Autodesk Inventor part; units mm, degrees
ref_plane "YZ Plane" through (0, 0, 0) normal (1, 0, 0) x (0, 1, 0)
ref_plane "XZ Plane" through (0, 0, 0) normal (0, 1, 0) x (-1, 0, 0)
ref_plane "XY Plane" through (0, 0, 0) normal (0, 0, 1) x (1, 0, 0)
sketch "Sketch1" plane through (0, 0, 0) normal (0, 0, 1) x (1, 0, 0)
  line L0 (-17.23, 12.6) -> (17.23, 12.6)
  line L1 (17.23, 12.6) -> (17.23, -12.6)
  line L2 (17.23, -12.6) -> (-17.23, -12.6)
  line L3 (-17.23, -12.6) -> (-17.23, 12.6)
  point P0 (0, 0)
  dimension "d0" = 17.23
  dimension "d1" = 34.46
  dimension "d2" = 12.6
  dimension "d3" = 25.2
extrude "Plate1" add sketch "Sketch1" along normal blind 0.5
sketch "Sketch4" plane through (-16.73, -12.6, 0) normal (-1, 0, 0) x (0, -1, 0)
  line L0 (-25.2, 0) -> (0, 0)
  line L1 (0, 0) -> (0, 8.75)
  line L2 (0, 8.75) -> (-25.2, 8.75)
  line L3 (-25.2, 8.75) -> (-25.2, 0)
edge flange "Flange1" height 8.75 angle 90 thickness 0.5 bend radius 0.5 thickness toward (-1, 0, 0) relief straight relief width 0.5 relief depth 0.25 edges at (-17.23, 0, 0.5) wall of the first edge with corners at (-16.73, 12.6, 0) (-16.73, -12.6, 0) (-16.73, -12.6, 8.75) (-16.73, 12.6, 8.75)
bend "Bend1"
corner "Corner1"
sketch "Sketch5" plane through (16.73, 12.6, 0) normal (1, 0, 0) x (0, 1, 0)
  line L0 (-25.2, 0) -> (0, 0)
  line L1 (0, 0) -> (0, 8.75)
  line L2 (0, 8.75) -> (-25.2, 8.75)
  line L3 (-25.2, 8.75) -> (-25.2, 0)
edge flange "Flange2" height 8.75 angle 90 thickness 0.5 bend radius 0.5 thickness toward (1, 0, 0) relief straight relief width 0.5 relief depth 0.25 edges at (17.23, 0, 0.5) wall of the first edge with corners at (16.73, -12.6, 0) (16.73, 12.6, 0) (16.73, 12.6, 8.75) (16.73, -12.6, 8.75)
bend "Bend2"
corner "Corner2"
sketch "Sketch6" plane through (0, 0, 0.5) normal (0, 0, 1) x (1, 0, 0)
  circle A0 centre (0, 0) radius 4
  circle A1 centre (0, 8.04) radius 1.65
  circle A2 centre (0, -8.04) radius 1.65
  circle A3 centre (8.04, 0) radius 1.65
  circle A4 centre (-8.04, 0) radius 1.65
  line L0 (16.23, -12.6) -> (-16.23, -12.6)
  line L1 (-16.23, 12.6) -> (16.23, 12.6)
  dimension "d26" = 3.3
  dimension "d27" = 8
  dimension "d29" = 4.56
  dimension "d30" = 4.56
  dimension "d31" = 8.04
  dimension "d32" = 8.04
  dimension "d33" = 8.04
extrude "Extrusion1" cut sketch "Sketch6" against normal through all
sketch "Sketch7" plane through (0, 0, 0.5) normal (0, 0, 1) x (1, 0, 0)
  circle A0 centre (0, 8.04) radius 1.65
  circle A1 centre (-8.04, 0) radius 1.65
  circle A2 centre (-8.04, 8.04) radius 1.6
  line L0 (0, -17.64) -> (0, 17.64)
  line L1 (-24.122, 0) -> (24.122, 0)
  circle A3 centre (8.04, 8.04) radius 1.6
  circle A4 centre (-8.04, -8.04) radius 1.6
  circle A5 centre (8.04, -8.04) radius 1.6
  point P0 (0, 0)
  dimension "d36" = 3.2
extrude "Extrusion2" cut sketch "Sketch7" against normal through all contours A2 | A3 | A4 | A5
sketch "Sketch8" plane through (0, 0, 0.5) normal (0, 0, 1) x (1, 0, 0)
  circle A0 centre (-8.04, 8.04) radius 1.6
  circle A1 centre (8.04, 8.04) radius 1.6
  circle A2 centre (8.04, -8.04) radius 1.6
  circle A3 centre (-8.04, -8.04) radius 1.6
  circle A4 centre (-8.04, 8.04) radius 3.1
  circle A5 centre (8.04, 8.04) radius 3.1
  circle A6 centre (8.04, -8.04) radius 3.1
  circle A7 centre (-8.04, -8.04) radius 3.1
  point P0 (0, 0)
  dimension "d39" = 6.2
extrude "Extrusion3" add sketch "Sketch8" along normal blind 2.28
thread "Thread1"
thread "Thread2"
thread "Thread3"
thread "Thread4"
sketch "Sketch9" plane through (-17.23, -12.6, 8.75) normal (-1, 0, 0) x (0, 0, 1)
  circle A0 centre (-3.5174, 20.57) radius 1.2
  circle A1 centre (-2.9878, 4.57) radius 1.2
  line L0 (-7.75, 25.2) -> (0, 25.2)
  point P0 (-8.75, 12.6)
  dimension "d50" = 2.4
  dimension "d51" = 16
  dimension "d52" = 4.63
extrude "Extrusion4" cut sketch "Sketch9" against normal through all
equation "\"d30\" = d29"
equation "\"d6\" = BendReliefWidth"
equation "\"d7\" = BendReliefDepth"
equation "\"d8\" = MinimumRemnant"
equation "\"d9\" = BendRadius"
equation "\"d12\" = BendRadius"
equation "\"d13\" = CornerReliefSize"
equation "\"d14\" = GapSize"
equation "\"d15\" = JacobiRadiusSize"
equation "\"d16\" = BendReliefWidth"
equation "\"d17\" = BendReliefDepth"
equation "\"d18\" = MinimumRemnant"
equation "\"d19\" = BendRadius"
equation "\"d22\" = BendRadius"
equation "\"d23\" = CornerReliefSize"
equation "\"d24\" = GapSize"
equation "\"d25\" = JacobiRadiusSize"
equation "\"BendRadius\" = Thickness"
equation "\"BendReliefWidth\" = Thickness"
equation "\"BendReliefDepth\" = 0.5 * Thickness"
equation "\"CornerReliefSize\" = 4 * Thickness"
equation "\"MinimumRemnant\" = 2 * Thickness"
equation "\"TransitionRadius\" = BendRadius"
equation "\"JacobiRadiusSize\" = Thickness"
equation "\"GapSize\" = Thickness"
equation "\"d4\" = BendRadius"
properties part number "Servo Bracket"
Verification items for the finished model (mm, model axes). A direction names the side the tool comes from. Coordinates: 2 decimals unless noted, no trailing zeros. Order: outer loops, then holes, each group sorted by start corner. A loop starts at its lowest first (then second) coordinate and runs counter-clockwise, first axis right, second up. Notation, with made-up numbers: (31, 40) -> (81, 40) arc R17 cw to (81, 53) -> close; hole circle Ø11 at (14, 52.5). An arc over 180 degrees is marked (long way). Answer as CSV lines item,"result". Start each with the question number.
1) Cross-section at A-A, the plane z = 2.25. Give the number of separate pieces and of enclosed holes in the cut face, then the cut area to 3 significant figures.
2) Release check for a two-part mould opening along X. For faces 1 (the face through (-0.867, -3.905, 0.254)), 2 (the face through (-0.215, 9.676, 0.254)), 3 (the face through (0.1, -12.6, 0.2)), 4 (the face through (-16.945, -0.176, 0.301)) record: released by +X, released by -X, zero draft, split by the parting line, or undercut.
3) Gauge pin test, flat ends, axial feed: pin 1 Ø4 at (x, z) = (8.5, 3) entering from +Y; pin 2 Ø5.5 at (x, y) = (-8.04, 0) entering from +Z; pin 3 Ø3 at (x, y) = (9, 8.5) entering from +Z; pin 4 Ø2 at (x, y) = (0, 8.04) entering from +Z. Record the tip position at first contact, or that the pin passes through.
4) Cross-section at D-D, the plane x = -8.04. Record the boundary of the cut face in (y, z).
5) Material ranges on L1, parallel to Y at x = 8.04, z = 1.7; L2, parallel to X at y = 10.75, z = 2.25; L3, parallel to X at y = -9.5, z = 2, recorded low to high. Write a range as [from, to].
6) Cross-section at B-B, the plane x = 0. Record the boundary of the cut face in (y, z), then the cut area to 3 significant figures.
7) Cross-section at C-C, the plane y = 2.5. Record the boundary of the cut face in (x, z).
8) Set-up check for faces 5 (the face through (-6.37, -10.65, 1.62)), 6 (the face through (-9.69, 0.07, 0.25)), 7 (the face through (-6.7, -9.4, 2.78)): record each of +Z, -Z, +X, -X, +Y, -Y from which the full face is reachable in a straight line by a thin tool's end or side.
Conclusion:
1,separate pieces,"6"
1,enclosed holes,"4"
1,area,"114 mm²"
2,face 1,"undercut"
2,face 2,"undercut"
2,face 3,"zero draft"
2,face 4,"released by -X"
3,pin 1,"stops at y = 11.14"
3,pin 2,"stops at z = 0.5"
3,pin 3,"stops at z = 2.78"
3,pin 4,"passes through"
4,outline,"(-12.6, 0) -> (-9.64, 0) -> (-9.64, 2.78) -> (-11.14, 2.78) -> (-11.14, 0.5) -> (-12.6, 0.5) -> close; (-6.44, 0) -> (-1.65, 0) -> (-1.65, 0.5) -> (-4.94, 0.5) -> (-4.94, 2.78) -> (-6.44, 2.78) -> close; (1.65, 0) -> (6.44, 0) -> (6.44, 2.78) -> (4.94, 2.78) -> (4.94, 0.5) -> (1.65, 0.5) -> close; (9.64, 0) -> (12.6, 0) -> (12.6, 0.5) -> (11.14, 0.5) -> (11.14, 2.78) -> (9.64, 2.78) -> close"
5,L1,"y = [-11.14, -9.64], [-6.44, -4.94], [4.94, 6.44], [9.64, 11.14]"
5,L2,"x = [-17.23, -16.73], [-9.55, -6.53], [6.53, 9.55], [16.73, 17.23]"
5,L3,"x = [-17.23, -16.73], [-10.77, -8.69], [-7.39, -5.31], [5.31, 7.39], [8.69, 10.77], [16.73, 17.23]"
6,outline,"(-12.6, 0) -> (-9.69, 0) -> (-9.69, 0.5) -> (-12.6, 0.5) -> close; (-6.39, 0) -> (-4, 0) -> (-4, 0.5) -> (-6.39, 0.5) -> close; (4, 0) -> (6.39, 0) -> (6.39, 0.5) -> (4, 0.5) -> close; (9.69, 0) -> (12.6, 0) -> (12.6, 0.5) -> (9.69, 0.5) -> close"
6,area,"5.30 mm²"
7,outline,"(-17.23, 1) arc R1 ccw to (-16.23, 0) -> (-3.12, 0) -> (-3.12, 0.5) -> (-16.23, 0.5) arc R0.5 cw to (-16.73, 1) -> (-16.73, 8.75) -> (-17.23, 8.75) -> close; (3.12, 0) -> (16.23, 0) arc R1 ccw to (17.23, 1) -> (17.23, 8.75) -> (16.73, 8.75) -> (16.73, 1) arc R0.5 cw to (16.23, 0.5) -> (3.12, 0.5) -> close"
8,face 5,"+Z"
8,face 6,"+Z, -Z"
8,face 7,"+Z, +Y, -Y"
